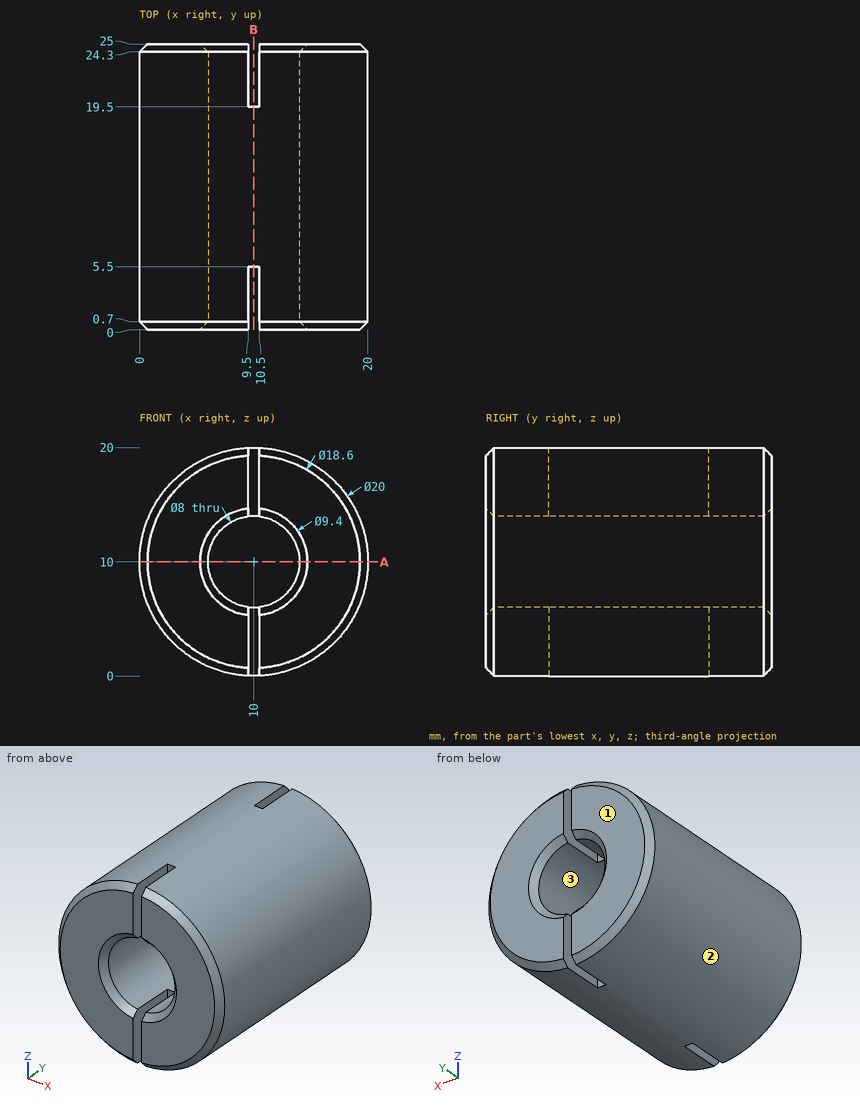
Here's the drawing with two shaded views (mm, measured from the low corner). I have some questions. Coordinates: 2 decimals unless noted, no trailing zeros. Write each loop counter-clockwise with the first axis right and the second up, starting at its lowest first coordinate (ties: lowest second). Pieces come first, ordered by that corner, then holes. Notation, with made-up numbers: M 26,33.5 L 66,33.5 A15 cw 66,55.5 Z; hole C 88.5,80 d5. An arc over 180 degrees is marked long. Answer as CSV lines item,"result".
Item 1: Imagine slicing it at A-A on z = 10. List the corners of the cut face in (x, y) for me.
Geometry results:
outline,"M 0,0.7 L 0.7,0 L 5.3,0 L 6,0.7 L 6,24.3 L 5.3,25 L 0.7,25 L 0,24.3 Z; M 14,0.7 L 14.7,0 L 19.3,0 L 20,0.7 L 20,24.3 L 19.3,25 L 14.7,25 L 14,24.3 Z"
Item 2: Imagine slicing it at B-B on x = 10. List the corners of the cut face in (y, z) for me, plus the area to 3 significant figures.
Geometry results:
outline,"M 5.5,0 L 19.5,0 L 19.5,6 L 5.5,6 Z; M 5.5,14 L 19.5,14 L 19.5,20 L 5.5,20 Z"
area,"168 mm2"
Item 3: We'd pull the mould along Z, two halves only. Please class the marked faces 1, 2 and 3: +Z half, -Z half, draft (parallel to the pull), parting line (faces both ways), or undercut.
Geometry results:
face 1,"draft"
face 2,"parting line"
face 3,"undercut"
Item 4: I'm going to push flat-ended pins straight in: P1, Ø1.5, axis at x = 14.5, y = 10.5, coming from the -Z side; P2, Ø5, axis at y = 6, z = 16.5, coming from the +X side; P3, Ø0.5, axis at x = 10, z = 18, coming from the -Y side. Where does each tip first touch, or does it pass through?
Geometry results:
P1,"stops at z = 0.73"
P2,"stops at x = 19.17"
P3,"stops at y = 5.5"
Item 5: Please list where these lines run through material, in increasing order: line 1 along X through (y, z) = (6.25, 10); line 2 along X through (y, z) = (2, 3.75).
Geometry results:
line 1,"x = 0 to 6, 14 to 20"
line 2,"x = 2.19 to 9.5, 10.5 to 17.81"
